```python
from build123d import *

# Parameters (mm, degrees)
CUT_EXTRUDE_START    = -195
CUT_EXTRUDE_3_DEPTH  = 5
SKETCH_33_R          = 1.6
CUT_EXTRUDE_6_DEPTH  = 10
CUT_EXTRUDE_START_2  = -10
CUT_EXTRUDE_21_DEPTH = 60


with BuildPart() as part:
    # 草图24 → 旋转4 (revolve)
    with BuildSketch(Plane.XY):
        Polygon((-45.743520691, 338.209134615), (-21.309763961, 338.209134615), (-21.309763961, 138.209134615), (-45.743520691, 138.209134615), (-31.309763961, 163.209134615), (-31.309763961, 313.209134615), align=None)
    revolve(axis=Axis((-21.309763961, 338.209134615, 0), (0, -1, 0)))

    # 草图29 → 切除-拉伸3 (cut)
    with BuildSketch(Plane(origin=(0, 338.209134615, 0), x_dir=(1, 0, 0), z_dir=(0, 1, 0)).offset(CUT_EXTRUDE_START)):
        Polygon((-21.309763961, 0), (-19.510610987, 7.281006014), (-42.085820567, 12.859391114), align=None)
        with BuildLine():
            ThreePointArc((3.123992769, 0), (3.109139711, 0.851828276), (3.064598594, 1.702620914))
            Line((3.064598594, 1.702620914), (-21.309763961, 0))
            Line((-21.309763961, 0), (-0.533707355, -12.859391114))
            ThreePointArc((-0.533707355, -12.859391114), (2.191784721, -6.684734662), (3.123992769, 0))
        make_face()
        with BuildLine():
            Line((-45.684126516, -1.702620914), (-21.309763961, 0))
            Line((-21.309763961, 0), (-42.085820567, 12.859391114))
            ThreePointArc((-42.085820567, 12.859391114), (-45.030074587, 5.861342146), (-45.684126516, -1.702620914))
        make_face()
        Polygon((-23.108916935, -7.281006014), (-21.309763961, 0), (-45.684126516, -1.702620914), align=None)
        Polygon((-21.309763961, 0), (3.064598594, 1.702620914), (-19.510610987, 7.281006014), align=None)
        Polygon((-0.533707355, -12.859391114), (-21.309763961, 0), (-23.108916935, -7.281006014), align=None)
    extrude(amount=-CUT_EXTRUDE_3_DEPTH, mode=Mode.SUBTRACT)

    # 草图33 → 切除-拉伸6 (cut)
    with BuildSketch(Plane.XZ.offset(-143.209134615)):
        with Locations(Location((-28.909264197, -1.519900047, 0), (0, 0, 270))):
            Circle(SKETCH_33_R)
        with Locations(Location((-13.730491725, 1.619346078, 0), (0, 0, 270))):
            Circle(SKETCH_33_R)
    extrude(amount=-CUT_EXTRUDE_6_DEPTH, mode=Mode.SUBTRACT)

    # 草图35 → 切除-拉伸21 (cut)
    with BuildSketch(Plane.XZ.offset(-143.209134615).offset(CUT_EXTRUDE_START_2)):
        Polygon((-24.909264197, -1.519900047), (-26.909264197, 1.944201568), (-30.909264197, 1.944201568), (-32.909264197, -1.519900047), (-30.909264197, -4.984001662), (-26.909264197, -4.984001662), align=None)
        Polygon((-9.730491725, 1.619346078), (-11.730491725, 5.083447693), (-15.730491725, 5.083447693), (-17.730491725, 1.619346078), (-15.730491725, -1.844755537), (-11.730491725, -1.844755537), align=None)
    extrude(amount=-CUT_EXTRUDE_21_DEPTH, mode=Mode.SUBTRACT)


solid = part.part
```
For this review, take the finished solid that the model builds, in its own axes (mm). A direction names the side the tool comes from. Give positions to 0.01 mm unless a question says otherwise; leave off trailing zeros. Write each loop counter-clockwise with the first axis right and the second up, starting at its lowest first coordinate (ties: lowest second). Pieces come first, ordered by that corner, then holes.
Item 1: Wall thickness on probe 1 along Z at (x, y) = (-29, 160); probe 2 along Y at (x, z) = (-9.5, 2); probe 3 along Y at (x, z) = (-42, 6.5): over which ranges is each line inside the solid? List them lowest first.
Item 2: Insertion check: P1, Ø12, axis at x = -26.5, y = 249.5, coming from the +Z side; P2, Ø4, axis at y = 178, z = -8.5, coming from the +X side; P3, Ø1.2, axis at x = -13, y = 171, coming from the -Z side; P4, Ø3, axis at y = 212.5, z = -12.5, coming from the +X side. Each pin has a flat end and moves straight along its axis. Give the tip position at first contact, or say it passes through.
Item 3: Take a section at B-B (y = 278.5). Give the boundary of the cut face in (x, z), and give its area (3 significant figures).
Item 4: Take a section at A-A (y = 202.5). Give the boundary of the cut face in (x, z), and give its area (3 significant figures).
Item 5: Machinability: for faces 1 (the face through (-12.144, 148.139, 1.828)), 2 (the face through (-29, 183, 1.944)), which of the approach directions +Z, -Z, +X, -X, +Y, -Y give a long, thin tool a straight path to every point of the face, cutting with its end or side? Answer none if there is none.
Item 6: The part is to be moulded in two halves that separate along Z. For faces 3 (the face through (-27, 153.209, -1)), 4 (the face through (-23, 138.209, 15)), 5 (the face through (-19.14, 239.26, 9.76)), say which applies: +Z half, -Z half, draft (parallel to the pull), parting line (faces both ways), or undercut.
Established:
1. probe 1: z = -9.02 to -4.98, 1.94 to 9.02
1. probe 2: y = 143.21 to 159.78, 316.63 to 338.21
1. probe 3: y = 138.21 to 142.97, 333.45 to 338.21
2. P1: stops at z = 10
2. P2: stops at x = -13.71
2. P3: stops at z = -6.37
2. P4: passes through
3. outline: circle Ø20 at (-21.31, 0)
3. area: 314 mm2
4. outline: (-31.21, 1.43) - (-30.91, 1.94) - (-26.91, 1.94) - (-24.91, -1.52) - (-26.91, -4.98) - (-29.98, -4.98) arc R10 ccw to (-11.39, -1.25) - (-11.73, -1.84) - (-15.73, -1.84) - (-17.73, 1.62) - (-15.73, 5.08) - (-12.7, 5.08) arc R10 ccw to start
4. area: 244 mm2
5. face 1: -Y
5. face 2: none
6. face 3: undercut
6. face 4: draft
6. face 5: parting line
